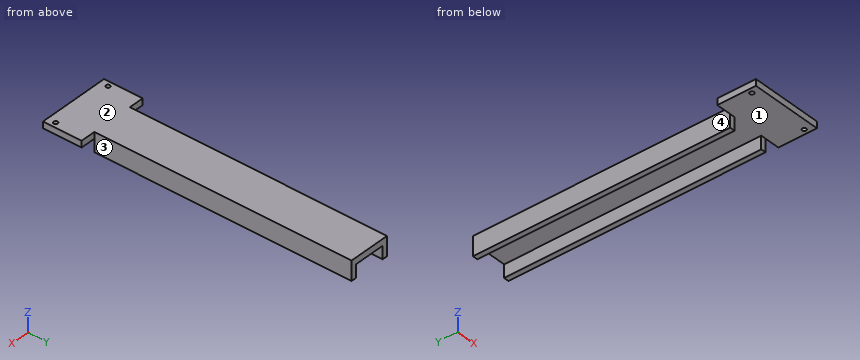
```python
from build123d import *

# Parameters (mm, degrees)
BOSS_EXTRUDE1_DEPTH            = 200
BOSS_EXTRUDE2_DEPTH            = 5
M3_CLEARANCE_HOLE1_D           = 3.2
M3_CLEARANCE_HOLE1_CSINK_D     = 3.25
M3_CLEARANCE_HOLE1_CSINK_ANGLE = 90


with BuildPart() as part:
    # Sketch1 → Boss-Extrude1 (new body)
    with BuildSketch(Plane(origin=(0, 0, 0), x_dir=(1, 0, 0), z_dir=(0, 1, 0))):
        Polygon((0, 0), (0, -15), (32.5, -15), (32.5, 0), (28.5, 0), (28.5, -10), (4, -10), (4, 0), align=None)
    extrude(amount=BOSS_EXTRUDE1_DEPTH)

    # Sketch2 → Boss-Extrude2 (add)
    with BuildSketch(Plane.XY.offset(15)):
        Polygon((32.5, 0), (44.25, 0), (44.25, -30), (-11.75, -30), (-11.75, 0), (0, 0), align=None)
    extrude(amount=-BOSS_EXTRUDE2_DEPTH)

    # M3 Clearance Hole1 (through all)
    with Locations(Plane(origin=(0, 0, 10), x_dir=(-1, 0, 0), z_dir=(0, 0, -1))):
        with Locations((7.75, -23.5), (-40.25, -23.5)):
            CounterSinkHole(M3_CLEARANCE_HOLE1_D / 2, M3_CLEARANCE_HOLE1_CSINK_D / 2, counter_sink_angle=M3_CLEARANCE_HOLE1_CSINK_ANGLE)


solid = part.part
```
Geometry check sheet. Reference: the model listing, model coordinates, mm. Face numbers are marked on the shaded views. Coordinates: 2 decimals unless noted, no trailing zeros. Loops run counter-clockwise (first coordinate to the right, second up) from the corner with the lowest first, then second, coordinate; pieces in that order, holes last.
Item 1: Sectioned sample at C-C, the plane x = 13.5. Record the boundary of the cut face in (y, z), then the cut area to 3 significant figures.
Item 2: Thickness scan on line 1 (X direction, y = -23.5, z = 13.35); line 2 (Y direction, x = 40.25, z = 13); line 3 (X direction, y = 182, z = 6.5). Record the ranges inside material, lowest first.
Item 3: Go/stop test with flat-tipped pins: pin 1 Ø3 at (y, z) = (123.5, 6.5) entering from +X; pin 2 Ø1.5 at (y, z) = (89.5, 2) entering from -X; pin 3 Ø5 at (x, y) = (33, 149) entering from -Z; pin 4 Ø4.5 at (x, z) = (3, 7) entering from -Y. Record where each tip stops, or that it passes through.
Item 4: Sectioned sample at A-A, the plane z = 5.25. Record the boundary of the cut face in (x, y), then the cut area to 3 significant figures.
Item 5: Sectioned sample at B-B, the plane y = 9. Record the boundary of the cut face in (x, z), then the cut area to 4 significant figures.
Item 6: Release check for a two-part mould opening along X. For the marked faces 1, 2, 3 and 4 record: released by +X, released by -X, zero draft, split by the parting line, or undercut.
Check result:
1. outline: (-30, 10) - (200, 10) - (200, 15) - (-30, 15) - close
1. area: 1,150 mm2
2. line 1: x = -11.75 to -9.35, -6.15 to 38.65, 41.85 to 44.25
2. line 2: y = -30 to -25.1, -21.9 to 0
2. line 3: x = 0 to 4, 28.5 to 32.5
3. pin 1: stops at x = 32.5
3. pin 2: stops at x = 0
3. pin 3: stops at z = 0
3. pin 4: stops at y = 0
4. outline: (0, 0) - (4, 0) - (4, 200) - (0, 200) - close; (28.5, 0) - (32.5, 0) - (32.5, 200) - (28.5, 200) - close
4. area: 1,600 mm2
5. outline: (0, 0) - (4, 0) - (4, 10) - (28.5, 10) - (28.5, 0) - (32.5, 0) - (32.5, 15) - (0, 15) - close
5. area: 242.5 mm2
6. face 1: undercut
6. face 2: zero draft
6. face 3: released by +X
6. face 4: released by -X
